For this review, take the finished solid that the model builds, in its own axes (mm). Face numbers are marked on the shaded views. A direction names the side the tool comes from. Round coordinates to 2 decimals unless told otherwise and drop trailing zeros. Order: outer loops, then holes, each group sorted by start corner. A loop starts at its lowest first (then second) coordinate and runs counter-clockwise, first axis right, second up. Notation, with made-up numbers: M 34.5,15 L 69.5,15 A12 cw 69.5,32 Z; hole C 20.5,-19.5 d9. An arc over 180 degrees is marked long. Put each result on its own line as item: value.
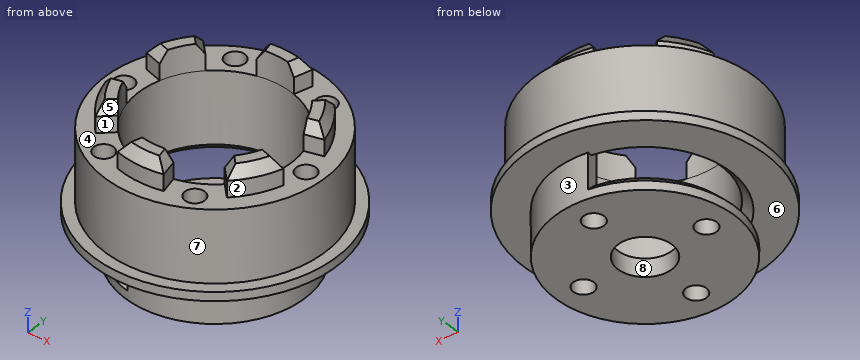
from build123d import *
from OCP.BRepFilletAPI import BRepFilletAPI_MakeChamfer

# Parameters (mm, degrees)
SKETCH_1_R          = 10
EXTRUDE_1_DEPTH     = 2
SKETCH_2_R          = 10
SKETCH_2_R_2        = 8.5
EXTRUDE_2_DEPTH     = 3
SKETCH_4_R          = 13.5
SKETCH_4_R_2        = 8.5
EXTRUDE_3_DEPTH     = 1
SKETCH_5_R          = 12.25
SKETCH_5_R_2        = 8.5
EXTRUDE_4_DEPTH     = 8
SKETCH_6_R          = 1.1
CUT_EXTRUDE_1_DEPTH = 8
SKETCH_7_R          = 3
SKETCH_7_R_2        = 1.15
CUT_EXTRUDE_2_DEPTH = 24.674881204
EXTRUDE_5_DEPTH     = 3
CHAMFER_1_SIZE      = 1.2
CHAMFER_1_SIZE2     = 0.840249046
CUT_EXTRUDE_START   = -2
CUT_EXTRUDE_3_DEPTH = 3
CHAMFER_2_SIZE      = 1


with BuildPart() as part:
    # 스케치1 → 보스-돌출1 (new body)
    with BuildSketch(Plane.XY):
        Circle(SKETCH_1_R)
    extrude(amount=EXTRUDE_1_DEPTH)

    # 스케치2 → 보스-돌출2 (add)
    with BuildSketch(Plane.XY.offset(2)):
        Circle(SKETCH_2_R)
        Circle(SKETCH_2_R_2, mode=Mode.SUBTRACT)
    extrude(amount=EXTRUDE_2_DEPTH)

    # 스케치4 → 보스-돌출3 (add)
    with BuildSketch(Plane.XY.offset(5)):
        Circle(SKETCH_4_R)
        Circle(SKETCH_4_R_2, mode=Mode.SUBTRACT)
    extrude(amount=EXTRUDE_3_DEPTH)

    # 스케치5 → 보스-돌출4 (add)
    with BuildSketch(Plane.XY.offset(6)):
        Circle(SKETCH_5_R)
        Circle(SKETCH_5_R_2, mode=Mode.SUBTRACT)
    extrude(amount=EXTRUDE_4_DEPTH)

    # 스케치6 → 컷-돌출1 (cut)
    with BuildSketch(Plane.XY.offset(14)):
        with Locations((10.375, 0)):
            Circle(SKETCH_6_R)
        with Locations((5.1875, -8.985013564)):
            Circle(SKETCH_6_R)
        with Locations((-5.1875, -8.985013564)):
            Circle(SKETCH_6_R)
        with Locations((-10.375, 0)):
            Circle(SKETCH_6_R)
        with Locations((-5.1875, 8.985013564)):
            Circle(SKETCH_6_R)
        with Locations((5.1875, 8.985013564)):
            Circle(SKETCH_6_R)
    extrude(amount=-CUT_EXTRUDE_1_DEPTH, mode=Mode.SUBTRACT)

    # 스케치7 → 컷-돌출2 (cut, through all)
    with BuildSketch(Plane(origin=(0, 0, 0), x_dir=(-1, 0, 0), z_dir=(0, 0, -1))):
        Circle(SKETCH_7_R)
        with Locations((-7, 0)):
            Circle(SKETCH_7_R_2)
        with Locations((7, 0)):
            Circle(SKETCH_7_R_2)
        with Locations((0, 7)):
            Circle(SKETCH_7_R_2)
        with Locations((0, -7)):
            Circle(SKETCH_7_R_2)
    extrude(amount=-CUT_EXTRUDE_2_DEPTH, mode=Mode.SUBTRACT)

    # 스케치10 → 보스-돌출5 (add)
    with BuildSketch(Plane.XY.offset(14)):
        with BuildLine():
            Line((-2.128230034, 8.229254943), (-2.628990043, 10.165550224))
            ThreePointArc((-2.628990043, 10.165550224), (0, 10.5), (2.628990043, 10.165550224))
            Line((2.628990043, 10.165550224), (2.128230034, 8.229254943))
            ThreePointArc((2.128230034, 8.229254943), (0, 8.5), (-2.128230034, 8.229254943))
        make_face()
        with BuildLine():
            Line((6.062628818, 5.957728747), (7.489129716, 7.359547275))
            ThreePointArc((7.489129716, 7.359547275), (9.09326674, 5.25), (10.118119759, 2.806002949))
            Line((10.118119759, 2.806002949), (8.190858852, 2.271526197))
            ThreePointArc((8.190858852, 2.271526197), (7.361215932, 4.25), (6.062628818, 5.957728747))
        make_face()
        with BuildLine():
            Line((-8.190858852, 2.271526197), (-10.118119759, 2.806002949))
            ThreePointArc((-10.118119759, 2.806002949), (-9.09326674, 5.25), (-7.489129716, 7.359547275))
            Line((-7.489129716, 7.359547275), (-6.062628818, 5.957728747))
            ThreePointArc((-6.062628818, 5.957728747), (-7.361215932, 4.25), (-8.190858852, 2.271526197))
        make_face()
        with BuildLine():
            Line((8.190858852, -2.271526197), (10.118119759, -2.806002949))
            ThreePointArc((10.118119759, -2.806002949), (9.09326674, -5.25), (7.489129716, -7.359547275))
            Line((7.489129716, -7.359547275), (6.062628818, -5.957728747))
            ThreePointArc((6.062628818, -5.957728747), (7.361215932, -4.25), (8.190858852, -2.271526197))
        make_face()
        with BuildLine():
            Line((2.128230034, -8.229254943), (2.628990043, -10.165550224))
            ThreePointArc((2.628990043, -10.165550224), (0, -10.5), (-2.628990043, -10.165550224))
            Line((-2.628990043, -10.165550224), (-2.128230034, -8.229254943))
            ThreePointArc((-2.128230034, -8.229254943), (0, -8.5), (2.128230034, -8.229254943))
        make_face()
        with BuildLine():
            Line((-6.062628818, -5.957728747), (-7.489129716, -7.359547275))
            ThreePointArc((-7.489129716, -7.359547275), (-9.09326674, -5.25), (-10.118119759, -2.806002949))
            Line((-10.118119759, -2.806002949), (-8.190858852, -2.271526197))
            ThreePointArc((-8.190858852, -2.271526197), (-7.361215932, -4.25), (-6.062628818, -5.957728747))
        make_face()
    extrude(amount=EXTRUDE_5_DEPTH)

    # 모따기1: one chamfer whose edges measure the first distance from different faces: ONE call of the kernel's chamfer builder (chamfer() names one face for all edges)
    chamfer_1_edges_1 = [part.edges().sort_by_distance(p)[0] for p in [
        (9.09326674, 5.25, 17),
    ]]
    chamfer_1_side_1 = [part.faces().sort_by_distance(p)[0] for p in [
        (9.09326674, 5.25, 15.5),
    ]]
    chamfer_1_edges_2 = [part.edges().sort_by_distance(p)[0] for p in [
        (6.775879267, 6.658638011, 17),
    ]]
    chamfer_1_side_2 = [part.faces().sort_by_distance(p)[0] for p in [
        (6.775879267, 6.658638011, 15.5),
    ]]
    chamfer_1_edges_3 = [part.edges().sort_by_distance(p)[0] for p in [
        (9.154489305, 2.538764573, 17),
    ]]
    chamfer_1_side_3 = [part.faces().sort_by_distance(p)[0] for p in [
        (9.154489305, 2.538764573, 15.5),
    ]]
    chamfer_1_edges_4 = [part.edges().sort_by_distance(p)[0] for p in [
        (-2.378610039, -9.197402584, 17),
    ]]
    chamfer_1_side_4 = [part.faces().sort_by_distance(p)[0] for p in [
        (-2.378610039, -9.197402584, 15.5),
    ]]
    chamfer_1_edges_5 = [part.edges().sort_by_distance(p)[0] for p in [
        (0, -10.5, 17),
    ]]
    chamfer_1_side_5 = [part.faces().sort_by_distance(p)[0] for p in [
        (0, -10.5, 15.5),
    ]]
    chamfer_1_edges_6 = [part.edges().sort_by_distance(p)[0] for p in [
        (2.378610039, -9.197402584, 17),
    ]]
    chamfer_1_side_6 = [part.faces().sort_by_distance(p)[0] for p in [
        (2.378610039, -9.197402584, 15.5),
    ]]
    chamfer_1_edges_7 = [part.edges().sort_by_distance(p)[0] for p in [
        (9.09326674, -5.25, 17),
    ]]
    chamfer_1_side_7 = [part.faces().sort_by_distance(p)[0] for p in [
        (9.09326674, -5.25, 15.5),
    ]]
    chamfer_1_edges_8 = [part.edges().sort_by_distance(p)[0] for p in [
        (9.154489305, -2.538764573, 17),
    ]]
    chamfer_1_side_8 = [part.faces().sort_by_distance(p)[0] for p in [
        (9.154489305, -2.538764573, 15.5),
    ]]
    chamfer_1_edges_9 = [part.edges().sort_by_distance(p)[0] for p in [
        (6.775879267, -6.658638011, 17),
    ]]
    chamfer_1_side_9 = [part.faces().sort_by_distance(p)[0] for p in [
        (6.775879267, -6.658638011, 15.5),
    ]]
    chamfer_1_edges_10 = [part.edges().sort_by_distance(p)[0] for p in [
        (2.378610039, 9.197402584, 17),
    ]]
    chamfer_1_side_10 = [part.faces().sort_by_distance(p)[0] for p in [
        (2.378610039, 9.197402584, 15.5),
    ]]
    chamfer_1_edges_11 = [part.edges().sort_by_distance(p)[0] for p in [
        (0, 10.5, 17),
    ]]
    chamfer_1_side_11 = [part.faces().sort_by_distance(p)[0] for p in [
        (0, 10.5, 15.5),
    ]]
    chamfer_1_edges_12 = [part.edges().sort_by_distance(p)[0] for p in [
        (-2.378610039, 9.197402584, 17),
    ]]
    chamfer_1_side_12 = [part.faces().sort_by_distance(p)[0] for p in [
        (-2.378610039, 9.197402584, 15.5),
    ]]
    chamfer_1_edges_13 = [part.edges().sort_by_distance(p)[0] for p in [
        (-6.775879267, 6.658638011, 17),
    ]]
    chamfer_1_side_13 = [part.faces().sort_by_distance(p)[0] for p in [
        (-6.775879267, 6.658638011, 15.5),
    ]]
    chamfer_1_edges_14 = [part.edges().sort_by_distance(p)[0] for p in [
        (-9.09326674, 5.25, 17),
    ]]
    chamfer_1_side_14 = [part.faces().sort_by_distance(p)[0] for p in [
        (-9.09326674, 5.25, 15.5),
    ]]
    chamfer_1_edges_15 = [part.edges().sort_by_distance(p)[0] for p in [
        (-9.154489305, 2.538764573, 17),
    ]]
    chamfer_1_side_15 = [part.faces().sort_by_distance(p)[0] for p in [
        (-9.154489305, 2.538764573, 15.5),
    ]]
    chamfer_1_edges_16 = [part.edges().sort_by_distance(p)[0] for p in [
        (-9.154489305, -2.538764573, 17),
    ]]
    chamfer_1_side_16 = [part.faces().sort_by_distance(p)[0] for p in [
        (-9.154489305, -2.538764573, 15.5),
    ]]
    chamfer_1_edges_17 = [part.edges().sort_by_distance(p)[0] for p in [
        (-9.09326674, -5.25, 17),
    ]]
    chamfer_1_side_17 = [part.faces().sort_by_distance(p)[0] for p in [
        (-9.09326674, -5.25, 15.5),
    ]]
    chamfer_1_edges_18 = [part.edges().sort_by_distance(p)[0] for p in [
        (-6.775879267, -6.658638011, 17),
    ]]
    chamfer_1_side_18 = [part.faces().sort_by_distance(p)[0] for p in [
        (-6.775879267, -6.658638011, 15.5),
    ]]
    chamfer_1 = BRepFilletAPI_MakeChamfer(part.part.solid().wrapped)
    for e in chamfer_1_edges_1:
        chamfer_1.Add(CHAMFER_1_SIZE, CHAMFER_1_SIZE2, e.wrapped, chamfer_1_side_1[0].wrapped)  # the first distance lies on this face
    for e in chamfer_1_edges_2:
        chamfer_1.Add(CHAMFER_1_SIZE, CHAMFER_1_SIZE2, e.wrapped, chamfer_1_side_2[0].wrapped)  # the first distance lies on this face
    for e in chamfer_1_edges_3:
        chamfer_1.Add(CHAMFER_1_SIZE, CHAMFER_1_SIZE2, e.wrapped, chamfer_1_side_3[0].wrapped)  # the first distance lies on this face
    for e in chamfer_1_edges_4:
        chamfer_1.Add(CHAMFER_1_SIZE, CHAMFER_1_SIZE2, e.wrapped, chamfer_1_side_4[0].wrapped)  # the first distance lies on this face
    for e in chamfer_1_edges_5:
        chamfer_1.Add(CHAMFER_1_SIZE, CHAMFER_1_SIZE2, e.wrapped, chamfer_1_side_5[0].wrapped)  # the first distance lies on this face
    for e in chamfer_1_edges_6:
        chamfer_1.Add(CHAMFER_1_SIZE, CHAMFER_1_SIZE2, e.wrapped, chamfer_1_side_6[0].wrapped)  # the first distance lies on this face
    for e in chamfer_1_edges_7:
        chamfer_1.Add(CHAMFER_1_SIZE, CHAMFER_1_SIZE2, e.wrapped, chamfer_1_side_7[0].wrapped)  # the first distance lies on this face
    for e in chamfer_1_edges_8:
        chamfer_1.Add(CHAMFER_1_SIZE, CHAMFER_1_SIZE2, e.wrapped, chamfer_1_side_8[0].wrapped)  # the first distance lies on this face
    for e in chamfer_1_edges_9:
        chamfer_1.Add(CHAMFER_1_SIZE, CHAMFER_1_SIZE2, e.wrapped, chamfer_1_side_9[0].wrapped)  # the first distance lies on this face
    for e in chamfer_1_edges_10:
        chamfer_1.Add(CHAMFER_1_SIZE, CHAMFER_1_SIZE2, e.wrapped, chamfer_1_side_10[0].wrapped)  # the first distance lies on this face
    for e in chamfer_1_edges_11:
        chamfer_1.Add(CHAMFER_1_SIZE, CHAMFER_1_SIZE2, e.wrapped, chamfer_1_side_11[0].wrapped)  # the first distance lies on this face
    for e in chamfer_1_edges_12:
        chamfer_1.Add(CHAMFER_1_SIZE, CHAMFER_1_SIZE2, e.wrapped, chamfer_1_side_12[0].wrapped)  # the first distance lies on this face
    for e in chamfer_1_edges_13:
        chamfer_1.Add(CHAMFER_1_SIZE, CHAMFER_1_SIZE2, e.wrapped, chamfer_1_side_13[0].wrapped)  # the first distance lies on this face
    for e in chamfer_1_edges_14:
        chamfer_1.Add(CHAMFER_1_SIZE, CHAMFER_1_SIZE2, e.wrapped, chamfer_1_side_14[0].wrapped)  # the first distance lies on this face
    for e in chamfer_1_edges_15:
        chamfer_1.Add(CHAMFER_1_SIZE, CHAMFER_1_SIZE2, e.wrapped, chamfer_1_side_15[0].wrapped)  # the first distance lies on this face
    for e in chamfer_1_edges_16:
        chamfer_1.Add(CHAMFER_1_SIZE, CHAMFER_1_SIZE2, e.wrapped, chamfer_1_side_16[0].wrapped)  # the first distance lies on this face
    for e in chamfer_1_edges_17:
        chamfer_1.Add(CHAMFER_1_SIZE, CHAMFER_1_SIZE2, e.wrapped, chamfer_1_side_17[0].wrapped)  # the first distance lies on this face
    for e in chamfer_1_edges_18:
        chamfer_1.Add(CHAMFER_1_SIZE, CHAMFER_1_SIZE2, e.wrapped, chamfer_1_side_18[0].wrapped)  # the first distance lies on this face
    add(Compound.cast(chamfer_1.Shape()), mode=Mode.REPLACE)

    # 스케치11 → 컷-돌출3 (cut)
    with BuildSketch(Plane(origin=(0, 0, 0), x_dir=(-1, 0, 0), z_dir=(0, 0, -1)).offset(CUT_EXTRUDE_START)):
        with BuildLine():
            Line((1.736481777, 9.84807753), (0.520944533, 2.954423259))
            ThreePointArc((0.520944533, 2.954423259), (2.298133329, 1.928362829), (3, 0))
            Line((3, 0), (5.85, 0))
            ThreePointArc((5.85, 0), (7, 1.15), (8.15, 0))
            Line((8.15, 0), (10, 0))
            ThreePointArc((10, 0), (7.660444431, 6.427876097), (1.736481777, 9.84807753))
        make_face()
        with BuildLine():
            ThreePointArc((3, 0), (2.298133329, -1.928362829), (0.520944533, -2.954423259))
            Line((0.520944533, -2.954423259), (1.736481777, -9.84807753))
            ThreePointArc((1.736481777, -9.84807753), (7.660444431, -6.427876097), (10, 0))
            Line((10, 0), (8.15, 0))
            ThreePointArc((8.15, 0), (7, -1.15), (5.85, 0))
            Line((5.85, 0), (3, 0))
        make_face()
    extrude(amount=-CUT_EXTRUDE_3_DEPTH, mode=Mode.SUBTRACT)

    # 모따기2
    chamfer_2_edges = [part.edges().sort_by_distance(p)[0] for p in [
        (-8.5, 0, 5),
        (-10, 0, 2),
    ]]
    chamfer(chamfer_2_edges, length=CHAMFER_2_SIZE)


solid = part.part
(1) Add section B-B on z = 15. Give the boundary of the cut face in (x, y).
A:
outline: M -10.12,-2.81 A10.5 ccw -7.49,-7.36 L -6.06,-5.96 A8.5 cw -8.19,-2.27 Z; M -10.12,2.81 L -8.19,2.27 A8.5 cw -6.06,5.96 L -7.49,7.36 A10.5 ccw Z; M -2.63,-10.17 A10.5 ccw 2.63,-10.17 L 2.13,-8.23 A8.5 cw -2.13,-8.23 Z; M -2.63,10.17 L -2.13,8.23 A8.5 cw 2.13,8.23 L 2.63,10.17 A10.5 ccw Z; M 6.06,-5.96 L 7.49,-7.36 A10.5 ccw 10.12,-2.81 L 8.19,-2.27 A8.5 cw Z; M 6.06,5.96 A8.5 cw 8.19,2.27 L 10.12,2.81 A10.5 ccw 7.49,7.36 Z
(2) Add section C-C on x = 7. Give the boundary of the cut face in (y, z).
A:
outline: M -11.54,5 L -7.14,5 L -7.14,0 L -1.15,0 L -1.15,2 L -4.82,2 L -4.82,17 L -5.7,17 L -6.88,15.8 L -6.88,14 L -10.05,14 L -10.05,6 L -11.54,6 Z; M 1.15,0 L 7.14,0 L 7.14,5 L 11.54,5 L 11.54,6 L 10.05,6 L 10.05,14 L 6.88,14 L 6.88,15.8 L 5.7,17 L 4.82,17 L 4.82,2 L 1.15,2 Z
(3) For the marked faces 1, 2, 3 and 4, list the 3-axis set-ups (+Z, -Z, +X, -X, +Y, -Y) from which the entire face can be reached by the end or side of a thin tool; tool diameter is ignored.
A:
face 1: +Z, -Y
face 2: +Z, +X, -Y
face 3: -Z
face 4: +Z
(4) Add section A-A on x = 0. State how many separate pieces and enclosed holes the cut face has, then the cut area to 3 significant figures.
A:
separate pieces: 4
enclosed holes: 0
area: 109 mm2
(5) Insertion check: pin 1 Ø10 at (x, y) = (-1.5, -8) entering from -Z; pin 2 Ø6 at (x, z) = (-10, 4.5) entering from +Y; pin 3 Ø10 at (y, z) = (7.5, 10.5) entering from +X; pin 4 Ø5 at (x, y) = (-0.5, 1) entering from +Z. Each pin has a flat end and moves straight along its axis. Give the tip position at first contact, or say it passes through.
A:
pin 1: stops at z = 0
pin 2: stops at y = 11.52
pin 3: stops at x = 12.41
pin 4: stops at z = 2
(6) To check wall thickness, follow L1, parallel to Y at x = 0, z = 0.45; L2, parallel to Y at x = 0, z = 11.75; L3, parallel to Z at x = 11.75, y = 2.25. State the ranges of each line that lie inside material, in increasing order.
A:
L1: y = -10 to -8.15, -5.85 to -3, 3 to 5.85, 8.15 to 10
L2: y = -12.25 to -8.5, 8.5 to 12.25
L3: z = 5 to 14
(7) Draft analysis for pull direction X (two halves, no side actions). For the marked faces 5, 6, 7 and 8, state which applies: released by +X, released by -X, zero draft, split by the parting line, or undercut.
A:
face 5: undercut
face 6: zero draft
face 7: split by the parting line
face 8: undercut
